Design review of the part shown in the three views and the two pictorial views. Dimensions are in mm from the part's minimum x, y and z. A direction names the side the tool comes from. Give positions to 0.01 mm unless a question says otherwise; leave off trailing zeros. Loops run counter-clockwise (first coordinate to the right, second up) from the corner with the lowest first, then second, coordinate; pieces in that order, holes last. Notation, with made-up numbers: (79, -25.5) - (101, -25.5) arc R11 cw to (101, -4.5) - close; hole circle Ø10 at (-17, -35). An arc over 180 degrees is marked (long way). Use CSV: the item, a comma, the result in double quotes. Start each with the question number.
1. For the marked faces 1 and 2, list the 3-axis set-ups (+Z, -Z, +X, -X, +Y, -Y) from which the entire face can be reached by the end or side of a thin tool; tool diameter is ignored.
2. Take a section at A-A on y = 3.5. Give the boundary of the cut face in (x, z).
3. Take a section at B-B on z = 1.5. Give the boundary of the cut face in (x, y).
4. Wall thickness on line 1 (X direction, y = 1.25, z = 4.25); line 2 (Z direction, x = 4.75, y = 1.1); line 3 (X direction, y = 3.25, z = 11.25): over which ranges is each line inside the solid? List them lowest first.
5. For pin 1 (1.2 mm diameter, centred on y = 2.5, z = 7, fed in from +X), flat-tipped, find the tip position at first contact; note if it passes through.
6. Take a section at C-C on x = 7.25. Give the boundary of the cut face in (y, z).
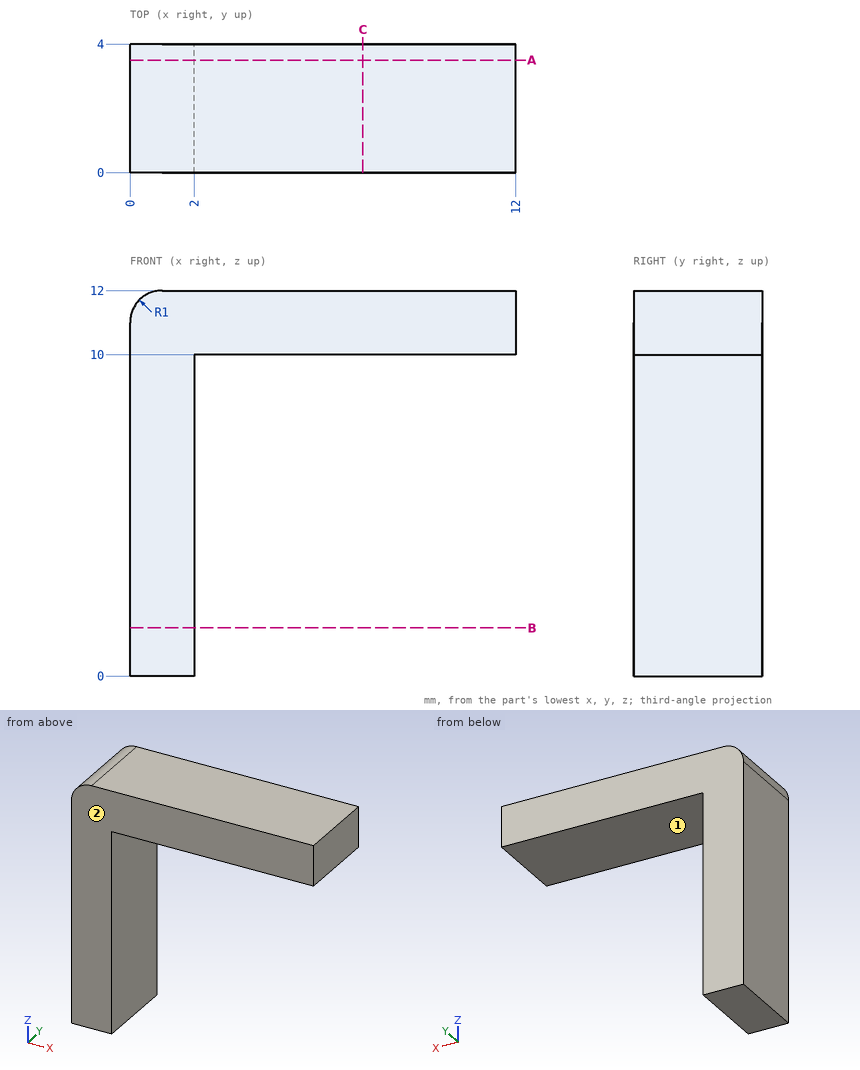
Check result:
1,face 1,"-Z, +X, +Y, -Y"
1,face 2,"+Z, -Z, +X, -X, -Y"
2,outline,"(0, 0) - (2, 0) - (2, 10) - (12, 10) - (12, 12) - (1, 12) arc R1 ccw to (0, 11) - close"
3,outline,"(0, 0) - (2, 0) - (2, 4) - (0, 4) - close"
4,line 1,"x = 0 to 2"
4,line 2,"z = 10 to 12"
4,line 3,"x = 0.03 to 12"
5,pin 1,"stops at x = 2"
6,outline,"(0, 10) - (4, 10) - (4, 12) - (0, 12) - close"
